Autodesk Inventor part; units mm, degrees
ref_plane "РабПлоскость1" through (-17.5, 0, 0) normal (1, 0, 0) x (0, 1, 0)
ref_plane "YZ Plane" through (0, 0, 0) normal (1, 0, 0) x (0, 1, 0)
ref_plane "XZ Plane" through (0, 0, 0) normal (0, 1, 0) x (-1, 0, 0)
sketch "Эскиз1" plane through (0, 0, 0) normal (0, 1, 0) x (-1, 0, 0)
  circle A0 centre (0, 0) radius 9.5
  line L0 (0, -9.5) -> (0, -17.5)
  arc A1 (-7.7, -15.715) -> (-7.7, 15.715) centre (0, 0) ccw
  line L1 (0, 9.5) -> (0, 17.5)
  point P0 (0, -10)
extrude "Выдавливание1" add sketch "Эскиз1" along normal blind 10 contours A0 L1 A1 L0
sketch "Эскиз2" plane through (0, 0, 17.5) normal (1, 0, 0) x (0, 0, -1)
  circle A0 centre (3.75, 5) radius 1.5
  circle A1 centre (31.25, 5) radius 1.5
  point P0 (17.5, 0)
extrude "Выдавливание2" cut sketch "Эскиз2" against normal through all
ref_plane "РабПлоскость1" through (-17.5, 0, 0) normal (1, 0, 0) x (0, 1, 0)
sketch "Эскиз3" plane through (-17.5, 0, 0) normal (1, 0, 0) x (0, 1, 0)
  line L0 (1, -17.25) -> (9, -17.25)
  line L1 (9, -17.25) -> (9, -10.25)
  line L2 (9, -10.25) -> (1, -10.25)
  line L3 (1, -10.25) -> (1, -17.25)
  circle A0 centre (5, -13.75) radius 1.5
  line L4 (1, -17.25) -> (9, -10.25) construction
  line L5 (9, -17.25) -> (1, -10.25) construction
  line L6 (1, 10.25) -> (9, 10.25)
  line L7 (9, 10.25) -> (9, 17.25)
  line L8 (9, 17.25) -> (1, 17.25)
  line L9 (1, 17.25) -> (1, 10.25)
  circle A1 centre (5, 13.75) radius 1.5
  line L10 (1, 10.25) -> (9, 17.25) construction
  line L11 (9, 10.25) -> (1, 17.25) construction
  point P0 (0, 0)
  dimension "d4" = 8
  dimension "d5" = 7
  dimension "d6" = 8
  dimension "d7" = 7
extrude "Выдавливание3" cut sketch "Эскиз3" along normal blind 10 contours L3 L2 L1 L0 | A0 | L9 L8 L7 L6 | A1
equation "\"d6\" = d4"
equation "\"d7\" = d5"
properties part number "000.402 - Зажим подшипника" material "Пластик АБС"
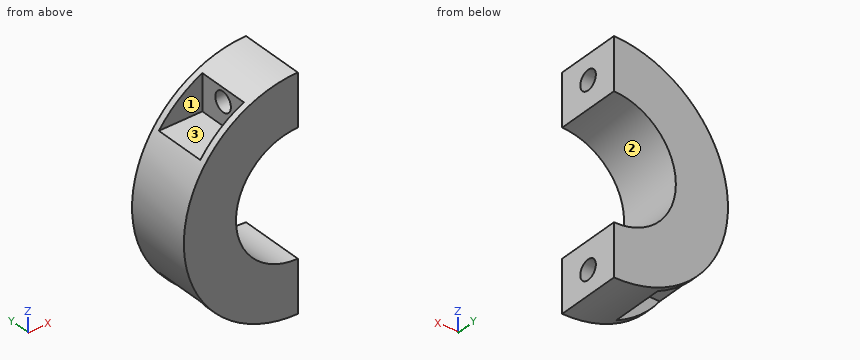
Model file for the job. Use its own axes, mm. Face numbers are marked on the shaded views. Coordinates: 2 decimals unless noted, no trailing zeros. Order: outer loops, then holes, each group sorted by start corner. A loop starts at its lowest first (then second) coordinate and runs counter-clockwise, first axis right, second up. Notation, with made-up numbers: (89.25, -16) -> (121.25, -16) arc R8 ccw to (121.25, -12) -> close; hole circle Ø7 at (45, -32.5). An arc over 180 degrees is marked (long way). Return JSON: item names as keys, results as strings.
Item 1: Wall check: line 1 along Y through (x, z) = (-3.5, -13.75); line 2 along X through (y, z) = (2.75, 12.5); line 3 along Z through (x, y) = (-4.5, 2.25). Give the ranges that are in metal, low to high. Write a range as from..to.
Model answer:
{"line 1": "y = 0..3.5, 6.5..10", "line 2": "x = -7.5..0", "line 3": "z = -16.91..-8.37, 8.37..16.91"}
Item 2: Pin check, flat tips, straight feed: P1, Ø1.8, axis at y = 5, z = 13.75, coming from the +X side; P2, Ø6, axis at x = -11.5, z = 13.5, coming from the -Y side; P3, Ø5, axis at x = -12, y = 5, coming from the +Z side; P4, Ø3, axis at y = 4, z = -10, coming from the -X side. Stop position of each tip, or through.
Model answer:
{"P1": "passes through", "P2": "stops at y = 0", "P3": "stops at z = 10.25", "P4": "stops at x = -15.3"}
Item 3: Slice it at D-D (y = 2.75). Write the cut outline in (x, z), then the cut area to 3 significant figures.
Model answer:
{"outline": "(-14.18, -10.25) -> (-7.5, -10.25) -> (-7.5, -15.81) arc R17.5 ccw to (0, -17.5) -> (0, -9.5) arc R9.5 cw to (0, 9.5) -> (0, 17.5) arc R17.5 ccw to (-7.5, 15.81) -> (-7.5, 10.25) -> (-14.18, 10.25) arc R17.5 ccw to start", "area": "296 mm²"}
Item 4: Mould opens along Z. For the marked faces 1, 2 and 3 say: pulls with the +Z half, pulls with the -Z half, needs draft (parallel to the pull), parting line crosses it, or undercut.
Model answer:
{"face 1": "needs draft", "face 2": "undercut", "face 3": "pulls with the +Z half"}
Item 5: Slice it at B-B (y = 5). Write the cut outline in (x, z), then the cut area to 3 significant figures.
Model answer:
{"outline": "(-14.18, -10.25) -> (-7.5, -10.25) -> (-7.5, -12.25) -> (0, -12.25) -> (0, -9.5) arc R9.5 cw to (0, 9.5) -> (0, 12.25) -> (-7.5, 12.25) -> (-7.5, 10.25) -> (-14.18, 10.25) arc R17.5 ccw to start; (-7.5, -15.81) arc R17.5 ccw to (0, -17.5) -> (0, -15.25) -> (-7.5, -15.25) -> close; (-7.5, 15.25) -> (0, 15.25) -> (0, 17.5) arc R17.5 ccw to (-7.5, 15.81) -> close", "area": "251 mm²"}
Item 6: Slice it at C-C (z = 13.75). Write the cut outline in (x, y).
Model answer:
{"outline": "(-10.83, 0) -> (0, 0) -> (0, 3.5) -> (-7.5, 3.5) -> (-7.5, 1) -> (-10.83, 1) -> close; (-10.83, 9) -> (-7.5, 9) -> (-7.5, 6.5) -> (0, 6.5) -> (0, 10) -> (-10.83, 10) -> close"}
Item 7: Slice it at A-A (x = -3.25). Write the cut outline in (y, z), then the cut area to 3 significant figures.
Model answer:
{"outline": "(0, -17.2) -> (10, -17.2) -> (10, -8.93) -> (0, -8.93) -> close; (0, 8.93) -> (10, 8.93) -> (10, 17.2) -> (0, 17.2) -> close; hole circle Ø3 at (5, -13.75); hole circle Ø3 at (5, 13.75)", "area": "151 mm²"}
